```python
from build123d import *

# Parameters (mm, degrees)
BOSS_EXTRUDE1_DEPTH = 95
SKETCH2_R           = 1.5
BOSS_EXTRUDE2_DEPTH = 2
SKETCH3_W           = 59.18
SKETCH3_H           = 25.4
CUT_EXTRUDE1_DEPTH  = 129.525100261


with BuildPart() as part:
    # Sketch1 → Boss-Extrude1 (new body)
    with BuildSketch(Plane.XY):
        Polygon((40.869322236, 66.889079057), (40.869322236, 30.389079057), (42.869322236, 30.389079057), (42.869322236, 31.389079057), (75.169322236, 31.389079057), (75.169322236, 65.889079057), (42.869322236, 65.889079057), (42.869322236, 66.889079057), align=None)
    extrude(amount=BOSS_EXTRUDE1_DEPTH)

    # Sketch2 → Boss-Extrude2 (add)
    # profile 1 of 2: a face of its own
    with BuildSketch(Plane.ZY.offset(-40.869322236)):
        with BuildLine():
            Line((-1, 38.389079057), (-8.25, 38.389079057))
            ThreePointArc((-8.25, 38.389079057), (-8.957106781, 38.096185839), (-9.25, 37.389079057))
            Line((-9.25, 37.389079057), (-9.25, 31.389079057))
            ThreePointArc((-9.25, 31.389079057), (-8.957106781, 30.681972276), (-8.25, 30.389079057))
            Line((-8.25, 30.389079057), (0, 30.389079057))
            Line((0, 30.389079057), (0, 38.389079057))
            Line((0, 38.389079057), (0, 66.889079057))
            Line((0, 66.889079057), (-1, 66.889079057))
            Line((-1, 66.889079057), (-1, 38.389079057))
        make_face()
        with Locations((-4.25, 34.389079057)):
            Circle(SKETCH2_R, mode=Mode.SUBTRACT)
    # profile 2 of 2: a face of its own
    with BuildSketch(Plane.ZY.offset(-40.869322236)):
        with BuildLine():
            Line((95, 66.889079057), (103.25, 66.889079057))
            ThreePointArc((103.25, 66.889079057), (103.957106781, 66.596185839), (104.25, 65.889079057))
            Line((104.25, 65.889079057), (104.25, 59.889079057))
            ThreePointArc((104.25, 59.889079057), (103.957106781, 59.181972276), (103.25, 58.889079057))
            Line((103.25, 58.889079057), (96, 58.889079057))
            Line((96, 58.889079057), (96, 30.389079057))
            Line((96, 30.389079057), (95, 30.389079057))
            Line((95, 30.389079057), (95, 58.889079057))
            Line((95, 58.889079057), (95, 66.889079057))
        make_face()
        with Locations((99.25, 62.889079057)):
            Circle(SKETCH2_R, mode=Mode.SUBTRACT)
    extrude(amount=-BOSS_EXTRUDE2_DEPTH)

    # Sketch3 → Cut-Extrude1 (cut, through all)
    with BuildSketch(Plane.ZY.offset(-40.869322236)):
        with Locations((47.49, 48.689079057)):
            Rectangle(SKETCH3_W, SKETCH3_H)
    extrude(amount=-CUT_EXTRUDE1_DEPTH, mode=Mode.SUBTRACT)


solid = part.part
```
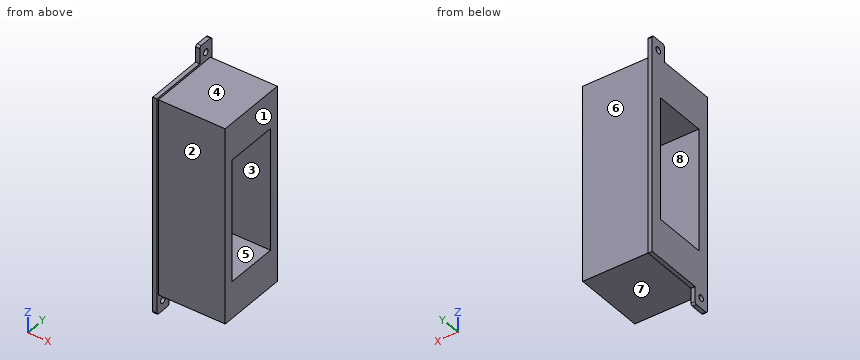
Could you check a few things on this model? Use its own coordinates, in mm. Face numbers are marked on the shaded views. A direction names the side the tool comes from. Round coordinates to 2 decimals unless told otherwise and drop trailing zeros. Loops run counter-clockwise (first coordinate to the right, second up) from the corner with the lowest first, then second, coordinate; pieces in that order, holes last. Notation, with made-up numbers: M 20.5,27 L 39.5,27 A28 cw 39.5,54 Z; hole C 29.25,60.5 d4. An arc over 180 degrees is marked long. Put each result on its own line as item: value.
Q1. Thinking about a two-plate mould opening in Z: for the marked faces 5, 6, 7 and 8, which applies, released by +Z, released by -Z, zero draft, split by the parting line, or undercut?
Check result:
face 5: undercut
face 6: zero draft
face 7: released by -Z
face 8: undercut
Q2. Imagine slicing it at D-D (z = 56). Write out the boundary of the cut face in (x, y).
Check result:
outline: M 40.87,30.39 L 42.87,30.39 L 42.87,31.39 L 75.17,31.39 L 75.17,35.99 L 40.87,35.99 Z; M 40.87,61.39 L 75.17,61.39 L 75.17,65.89 L 42.87,65.89 L 42.87,66.89 L 40.87,66.89 Z
Q3. Imagine slicing it at B-B (x = 73). Write out the boundary of the cut face in (y, z), then the cut area to 3 significant figures.
Check result:
outline: M 31.39,0 L 65.89,0 L 65.89,95 L 31.39,95 Z; hole M 35.99,17.9 L 61.39,17.9 L 61.39,77.08 L 35.99,77.08 Z
area: 1,770 mm2
Q4. I need wall thicknesses on probe 1 along Z at (x, y) = (73, 37); probe 2 along Y at (x, z) = (41.55, -4.25); probe 3 along Y at (x, z) = (66, 31). Which ranges of each line are inside material? Lowest first, please.
Check result:
probe 1: 0 to 17.9, 77.08 to 95
probe 2: 30.39 to 32.89, 35.89 to 38.39
probe 3: 31.39 to 35.99, 61.39 to 65.89
Q5. Imagine slicing it at A-A (z = -4.25). Write out the boundary of the cut face in (x, y), then the cut area to 4 significant figures.
Check result:
outline: M 40.87,30.39 L 42.87,30.39 L 42.87,32.89 L 40.87,32.89 Z; M 40.87,35.89 L 42.87,35.89 L 42.87,38.39 L 40.87,38.39 Z
area: 10.00 mm2
Q6. For pin 1 (6 mm diameter, centred on x = 48.5, y = 50.5, fed in from +Z); pin 2 (6 mm diameter, centred on x = 61.5, y = 35, fed in from -Z); pin 3 (1 mm diameter, centred on x = 60, z = 21, fed in from +Y); pin 4 (1.8 mm diameter, centred on y = 62.89, z = 99.25, fed in from -X), each with a flat end and sliding along its axis, tell me the tip position at first contact or that it passes through.
Check result:
pin 1: z = 95
pin 2: z = 0
pin 3: y = 65.89
pin 4: through
Q7. Imagine slicing it at C-C (y = 49). Write out the boundary of the cut face in (x, z), then the cut area to 3 significant figures.
Check result:
outline: M 40.87,-1 L 42.87,-1 L 42.87,0 L 75.17,0 L 75.17,17.9 L 40.87,17.9 Z; M 40.87,77.08 L 75.17,77.08 L 75.17,95 L 42.87,95 L 42.87,96 L 40.87,96 Z
area: 1,230 mm2
Q8. On a 3-axis mill with a long thin cutter (end or side, diameter ignored), from which of +Z, -Z, +X, -X, +Y, -Y can I reach the whole of each face in a straight line? I mean the marked faces 1, 2, 3 and 4. Say none if no direction works.
Check result:
face 1: +Z, -Z, +X, +Y, -Y
face 2: +Z, -Z, +X, -Y
face 3: +X, -X
face 4: +Z, +X, +Y, -Y
